Part print with two shaded views. Sizes in mm from the minimum x, y, z corner. Round coordinates to 2 decimals unless told otherwise and drop trailing zeros. Write each loop counter-clockwise with the first axis right and the second up, starting at its lowest first coordinate (ties: lowest second). Pieces come first, ordered by that corner, then holes. Notation, with made-up numbers: (57.5, 14.25) -> (94.5, 14.25) arc R15 ccw to (94.5, 39.25) -> close; hole circle Ø1 at (44.5, -11.75). An arc over 180 degrees is marked (long way). Answer as CSV lines item,"result".
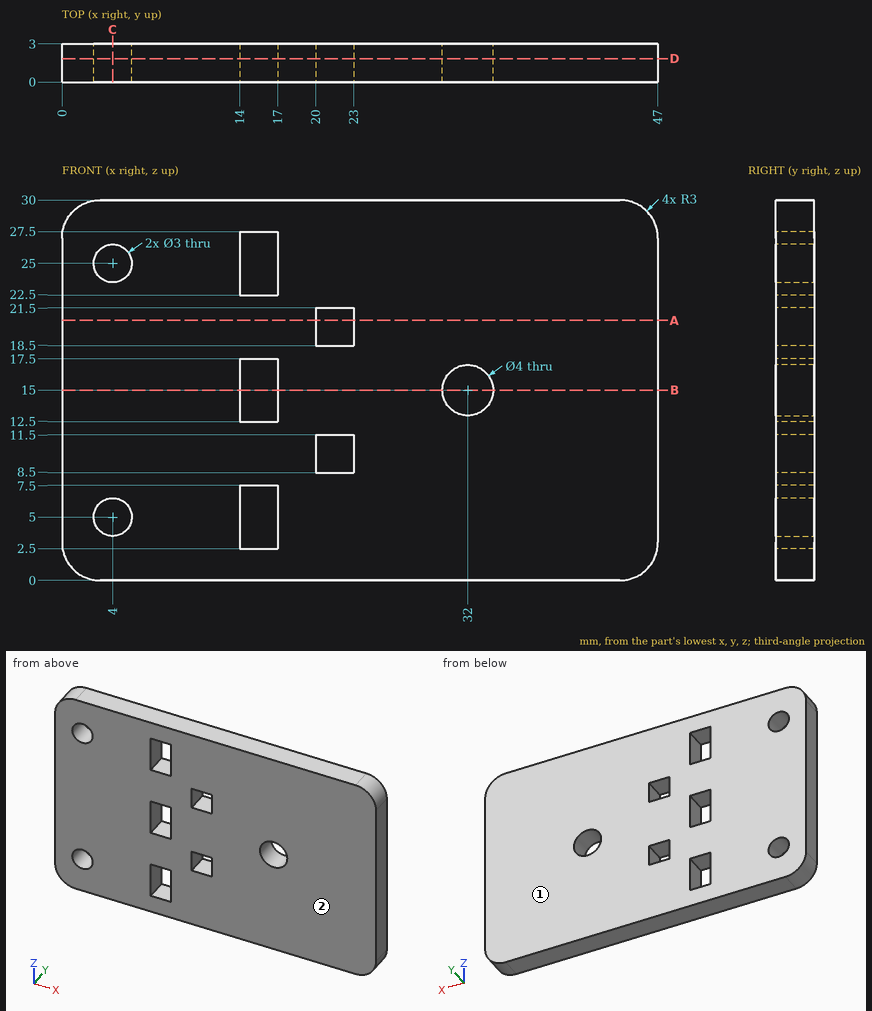
1. Cut at D-D, the plane y = 1.85. Count the separate pieces of the cut face and the enclosed holes in it, then the cut area to 3 significant figures.
Results found:
separate pieces,"1"
enclosed holes,"8"
area,"1,310 mm2"
2. Cut at B-B, the plane z = 15. Write the cut outline in (x, y).
Results found:
outline,"(0, 0) -> (14, 0) -> (14, 3) -> (0, 3) -> close; (17, 0) -> (30, 0) -> (30, 3) -> (17, 3) -> close; (34, 0) -> (47, 0) -> (47, 3) -> (34, 3) -> close"
3. Probe line 1 along Z through (x, y) = (22.5, 0.35); line 2 along X through (y, z) = (1.55, 15); line 3 along X through (y, z) = (1.35, 5). List the from-to ranges inside material, lowest first.
Results found:
line 1,"z = 0 to 8.5, 11.5 to 18.5, 21.5 to 30"
line 2,"x = 0 to 14, 17 to 30, 34 to 47"
line 3,"x = 0 to 2.5, 5.5 to 14, 17 to 47"
4. Mould opens along Y. For the marked faces 1 and 2 say: +Y half, -Y half, draft (parallel to the pull), parting line (faces both ways), or undercut.
Results found:
face 1,"+Y half"
face 2,"-Y half"
5. Cut at C-C, the plane x = 4. Write the cut outline in (y, z), then the cut area to 3 significant figures.
Results found:
outline,"(0, 0) -> (3, 0) -> (3, 3.5) -> (0, 3.5) -> close; (0, 6.5) -> (3, 6.5) -> (3, 23.5) -> (0, 23.5) -> close; (0, 26.5) -> (3, 26.5) -> (3, 30) -> (0, 30) -> close"
area,"72.0 mm2"
6. Cut at A-A, the plane z = 20.5. Write the cut outline in (x, y), then the cut area to 3 significant figures.
Results found:
outline,"(0, 0) -> (20, 0) -> (20, 3) -> (0, 3) -> close; (23, 0) -> (47, 0) -> (47, 3) -> (23, 3) -> close"
area,"132 mm2"
